Work out the finished part from the listing and answer in its coordinate system (mm). Face numbers are marked on the shaded views. A direction names the side the tool comes from. Coordinates: 2 decimals unless noted, no trailing zeros. Order: outer loops, then holes, each group sorted by start corner. A loop starts at its lowest first (then second) coordinate and runs counter-clockwise, first axis right, second up. Notation, with made-up numbers: (-3.75, 66.5) -> (43.25, 66.5) arc R27 ccw to (43.25, 103.5) -> close; hole circle Ø5 at (35.5, 48.5). An arc over 180 degrees is marked (long way). Use one line per item in the form item = value.
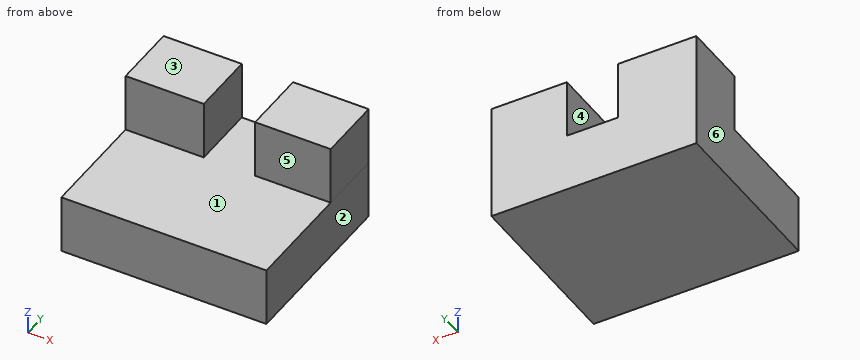
from build123d import *

# Parameters (mm, degrees)
F0_W     = 88.9
F0_H     = 76.2
F1_DEPTH = 25.4
F2_W     = 33.895806
F2_H     = 28.295222
F3_DEPTH = 25.4
F2_W_2   = 32.765687
F4_DEPTH = 25.4


with BuildPart() as f1:
    # F0 (on Top) → F1 (new body)
    with BuildSketch(Plane.XY):
        with Locations((1.73725, -6.644126)):
            Rectangle(F0_W, F0_H)
    extrude(amount=F1_DEPTH)

    # F2 (on face) → F3 (join)
    with BuildSketch(Plane.XY.offset(25.4)):
        with Locations((-25.764847, 17.308263)):
            Rectangle(F2_W, F2_H)
    extrude(amount=F3_DEPTH)

    # F2 (on face) → F4 (join)
    with BuildSketch(Plane.XY.offset(25.4)):
        with Locations((29.804406, 17.308263)):
            Rectangle(F2_W_2, F2_H)
    extrude(amount=F4_DEPTH)


solid = f1.part
(1) The mould has two halves that part along X. Classify the marked faces 1, 2 and 3: released by +X, released by -X, zero draft, split by the parting line, or undercut.
Data:
face_1 = undercut
face_2 = released by +X
face_3 = zero draft
(2) Section B-B on y = 18.5 is taken. Write down the section's boundary in (x, z).
Data:
outline = (-42.71, 0) -> (46.19, 0) -> (46.19, 50.8) -> (13.42, 50.8) -> (13.42, 25.4) -> (-8.82, 25.4) -> (-8.82, 50.8) -> (-42.71, 50.8) -> close
(3) Each of these flat-tipped pins is pushed along its axis until it touches: P1, Ø10, axis at x = 27, y = -34.5, coming from the -Z side; P2, Ø7.5, axis at x = -26, z = 44, coming from the -Y side; P3, Ø6, axis at x = 0.5, y = -7, coming from the +Z side. Where does it stop, or does it pass through?
Data:
P1 = 0
P2 = 3.16
P3 = 25.4
(4) Straight lines are drawn through the part: line 1 along X through (y, z) = (17.5, 36.5); line 2 along Z through (x, y) = (24.5, -17.5); line 3 along Y through (x, z) = (-30.5, 42). For each, find the intervals that lie inside material, in ascending order.
Data:
line_1 = -42.71 to -8.82, 13.42 to 46.19
line_2 = 0 to 25.4
line_3 = 3.16 to 31.46
(5) Section D-D on y = -32 is taken. Write down the section's boundary in (x, z).
Data:
outline = (-42.71, 0) -> (46.19, 0) -> (46.19, 25.4) -> (-42.71, 25.4) -> close
(6) Which of the six approach directions +Z, -Z, +X, -X, +Y, -Y give full straight-line access (tool end or side, diameter ignored) to the marked faces 4, 5 and 6?
Data:
face_4 = +Z, +Y, -Y
face_5 = +Z, +X, -X, -Y
face_6 = +Z, -Z, -X, +Y, -Y
(7) Section C-C on x = -26.5 is taken. Write down the section's boundary in (y, z), plus the area to 3 significant figures.
Data:
outline = (-44.74, 0) -> (31.46, 0) -> (31.46, 50.8) -> (3.16, 50.8) -> (3.16, 25.4) -> (-44.74, 25.4) -> close
area = 2,650 mm²
(8) Section A-A on z = 36.5 is taken. Write down the section's boundary in (x, y).
Data:
outline = (-42.71, 3.16) -> (-8.82, 3.16) -> (-8.82, 31.46) -> (-42.71, 31.46) -> close; (13.42, 3.16) -> (46.19, 3.16) -> (46.19, 31.46) -> (13.42, 31.46) -> close
